Could you check a few things on this model? Use its own coordinates, in mm. Coordinates: 2 decimals unless noted, no trailing zeros. Loops run counter-clockwise (first coordinate to the right, second up) from the corner with the lowest first, then second, coordinate; pieces in that order, holes last. Notation, with made-up numbers: (75, 78.5) -> (82, 78.5) arc R16 ccw to (82, 107.5) -> close; hole circle Ø5 at (-30, 84.5). An arc over 180 degrees is marked (long way). One line per question, with ' | ' between items. Start each with the question number.
(1) Suppose I cut it at C-C (y = 0.6). Please give me the cut outline in (x, z), plus the area to 3 significant figures.
(2) Suppose I cut it at A-A (x = 0). Please give me the cut outline in (y, z), plus the area to 3 significant figures.
(3) Suppose I cut it at D-D (z = 6). Please give me the cut outline in (x, y), plus the area to 3 significant figures.
(4) I'm going to push a flat-ended pin straight in: pin 1 Ø1.2 at (x, z) = (-8.49, 8.49) entering from -Y. Where does the tip first touch, or does it pass through?
(5) If I drill on line 1 along Z through (x, y) = (0, 0.5); line 2 along X through (y, z) = (0.4, 5.5); line 3 along Z through (x, y) = (-9.25, 0.7), over which ranges is the centre line in solid material (lowest first)?
(6) Suppose I cut it at B-B (z = 11). Please give me the cut outline in (x, y), plus the area to 3 significant figures.
(7) If we mould it in two halves opening along X, with no side actions, what happens to faces 1 (the face through (-0.297, 0.493, 13.497)), 2 (the face through (10.518, 0.493, 5.37)), 3 (the face through (10.5, 0.5, 0))? For each: pulls with the +X half, pulls with the -X half, needs draft (parallel to the pull), parting line crosses it, or undercut.
```python
from build123d import *

# Parameters (mm, degrees)
SKETCH1_R               = 13.5
BOSS_EXTRUDE1_DEPTH     = 1
CUT_EXTRUDE1_DEPTH      = 20.118054294
CUT_EXTRUDE1_DEPTH_BACK = 20.118054294
SKETCH19_R              = 1
CUT_EXTRUDE2_DEPTH      = 20.118054294
CUT_EXTRUDE2_DEPTH_BACK = 20.118054294
SKETCH20_R              = 7.5
SKETCH21_W              = 65.874202484
SKETCH21_H              = 51.979273979
CUT_EXTRUDE3_DEPTH      = 20.118054294


with BuildPart() as part:
    # Sketch1 → Boss-Extrude1 (new body)
    with BuildSketch(Plane(origin=(0, 0, 0), x_dir=(1, 0, 0), z_dir=(0, 1, 0))):
        with Locations(Location((0, 0, 0), (0, 0, 270))):
            Circle(SKETCH1_R)
    extrude(amount=BOSS_EXTRUDE1_DEPTH)

    # Sketch19 → Cut-Extrude1 (cut, two sides: drawn at the far end of the back side and taken through both)
    with BuildSketch(Plane(origin=(0, 1, 0), x_dir=(1, 0, 0), z_dir=(0, 1, 0)).offset(-CUT_EXTRUDE1_DEPTH_BACK)):
        with Locations(Location((0, 11, 0), (0, 0, 270))):
            Circle(SKETCH19_R)
        with Locations(Location((9.526279442, 5.5, 0), (0, 0, 270))):
            Circle(SKETCH19_R)
        with Locations(Location((9.526279442, -5.5, 0), (0, 0, 270))):
            Circle(SKETCH19_R)
        with Locations(Location((0, -11, 0), (0, 0, 270))):
            Circle(SKETCH19_R)
        with Locations(Location((-9.526279442, -5.5, 0), (0, 0, 270))):
            Circle(SKETCH19_R)
        with Locations(Location((-9.526279442, 5.5, 0), (0, 0, 270))):
            Circle(SKETCH19_R)
        with Locations(Location((-8.485281374, -8.485281374, 0), (0, 0, 270))):
            Circle(SKETCH19_R)
    extrude(amount=CUT_EXTRUDE1_DEPTH + CUT_EXTRUDE1_DEPTH_BACK, mode=Mode.SUBTRACT)

    # Sketch20 → Cut-Extrude2 (cut, two sides: drawn at the far end of the back side and taken through both)
    with BuildSketch(Plane(origin=(0, 1, 0), x_dir=(1, 0, 0), z_dir=(0, 1, 0)).offset(-CUT_EXTRUDE2_DEPTH_BACK)):
        with Locations(Location((0, 0, 0), (0, 0, 270))):
            Circle(SKETCH20_R)
    extrude(amount=CUT_EXTRUDE2_DEPTH + CUT_EXTRUDE2_DEPTH_BACK, mode=Mode.SUBTRACT)

    # Sketch21 → Cut-Extrude3 (cut, through all)
    with BuildSketch(Plane.XY):
        with Locations((-3.816154381, 6.321647006)):
            Rectangle(SKETCH21_W, SKETCH21_H)
    extrude(amount=-CUT_EXTRUDE3_DEPTH, mode=Mode.SUBTRACT)


solid = part.part
```
Checks:
1) outline: (-13.5, 0) -> (-7.5, 0) arc R7.5 cw to (7.5, 0) -> (13.5, 0) arc R13.5 ccw to start; hole circle Ø2 at (-9.53, 5.5); hole circle Ø2 at (-8.49, 8.49); hole circle Ø2 at (0, 11); hole circle Ø2 at (9.53, 5.5) | area: 185 mm^2
2) outline: (0, 7.5) -> (1, 7.5) -> (1, 10) -> (0, 10) -> close; (0, 12) -> (1, 12) -> (1, 13.5) -> (0, 13.5) -> close | area: 4.00 mm^2
3) outline: (-12.09, 0) -> (-10.39, 0) -> (-10.39, 1) -> (-12.09, 1) -> close; (-8.66, 0) -> (-4.5, 0) -> (-4.5, 1) -> (-8.66, 1) -> close; (4.5, 0) -> (8.66, 0) -> (8.66, 1) -> (4.5, 1) -> close; (10.39, 0) -> (12.09, 0) -> (12.09, 1) -> (10.39, 1) -> close | area: 11.7 mm^2
4) pin 1: passes through
5) line 1: z = 7.5 to 10, 12 to 13.5 | line 2: x = -12.33 to -10.53, -8.53 to -5.1, 5.1 to 8.53, 10.53 to 12.33 | line 3: z = 0 to 4.54, 6.46 to 7.84, 9.13 to 9.83
6) outline: (-7.83, 0) -> (-1, 0) -> (-1, 1) -> (-7.83, 1) -> close; (1, 0) -> (7.83, 0) -> (7.83, 1) -> (1, 1) -> close | area: 13.7 mm^2
7) face 1: parting line crosses it | face 2: undercut | face 3: needs draft
